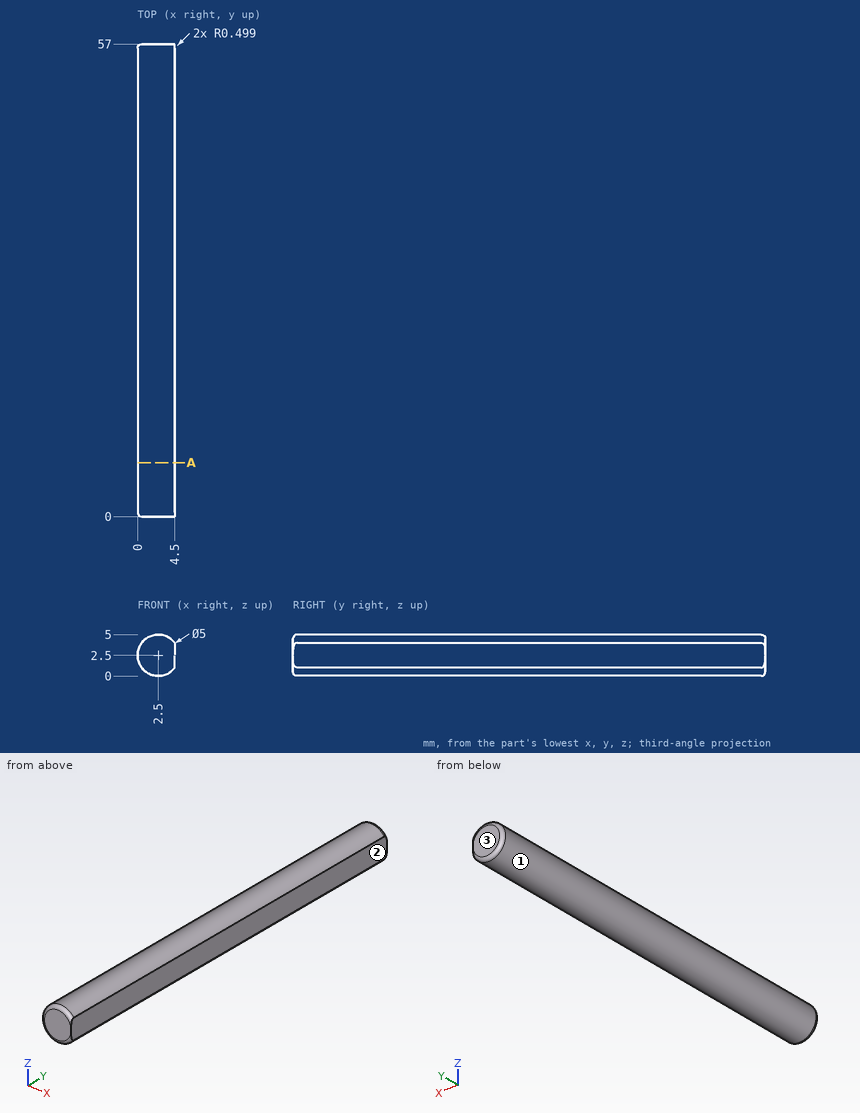
Design review of the part shown in the three views and the two pictorial views. Dimensions are in mm from the part's minimum x, y and z. Round coordinates to 2 decimals unless told otherwise and drop trailing zeros. Loops run counter-clockwise (first coordinate to the right, second up) from the corner with the lowest first, then second, coordinate; pieces in that order, holes last. Notation, with made-up numbers: M -23,57.5 L 22,57.5 A21 ccw 22,82.5 Z; hole C 88.5,85.25 d5. An arc over 180 degrees is marked long. Write item = value, one per line.
Item 1: The part is to be moulded in two halves that separate along X. For the marked faces 1, 2 and 3, say which applies: released by +X, released by -X, zero draft, split by the parting line, or undercut.
Return value:
face_1 = split by the parting line
face_2 = released by +X
face_3 = zero draft
Item 2: For line 1 (Z direction, x = 2.65, y = 44) (1 decimal); line 2 (X direction, y = 13, z = 2.3); line 3 (X direction, y = 20.5, z = 1.4) (1 decimal), list the stretches that pass through material, from the lowest coordinate up. Write a range as [from, to].
Return value:
line_1 = [0, 5]
line_2 = [0.01, 4.5]
line_3 = [0.3, 4.5]
Item 3: Take a section at A-A on y = 6.5. Write out the cut boundary in (x, z), then the cut area to 3 significant figures.
Return value:
outline = M 4.5,1 L 4.5,4 A2.5 ccw long Z
area = 18.6 mm2
